from build123d import *

# Parameters (mm, degrees)
SKETCH_1_R          = 4
EXTRUDE_1_DEPTH     = 10
SKETCH_2_R          = 2.6
CUT_EXTRUDE_1_DEPTH = 10


with BuildPart() as part:
    # 草图1 → 凸台-拉伸1 (new body)
    with BuildSketch(Plane.XY):
        with BuildLine():
            Line((-27.5, -15), (27.5, -15))
            Line((27.5, -15), (27.5, -9.7))
            Line((27.5, -9.7), (15, -9.7))
            Line((15, -9.7), (15, 0))
            ThreePointArc((15, 0), (0, 15), (-15, 0))
            Line((-15, 0), (-15, -9.7))
            Line((-15, -9.7), (-27.5, -9.7))
            Line((-27.5, -9.7), (-27.5, -15))
        make_face()
        Circle(SKETCH_1_R, mode=Mode.SUBTRACT)
    extrude(amount=EXTRUDE_1_DEPTH)

    # 草图2 → 切除-拉伸1 (cut)
    with BuildSketch(Plane(origin=(0, -9.7, 0), x_dir=(1, 0, 0), z_dir=(0, 1, 0))):
        with Locations((21, -5)):
            Circle(SKETCH_2_R)
        with Locations((-21, -5)):
            Circle(SKETCH_2_R)
    extrude(amount=-CUT_EXTRUDE_1_DEPTH, mode=Mode.SUBTRACT)


solid = part.part
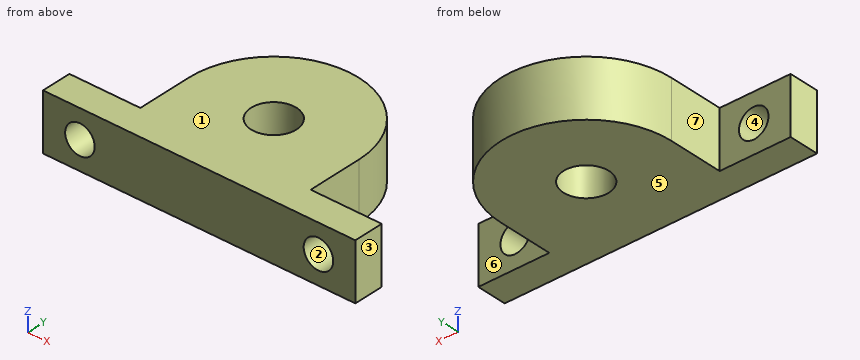
Here's how the part is built. I have some questions about the finished solid (model axes, mm). Face numbers are marked on the shaded views. A direction names the side the tool comes from. Give positions to 0.01 mm unless a question says otherwise; leave off trailing zeros. Order: outer loops, then holes, each group sorted by start corner. A loop starts at its lowest first (then second) coordinate and runs counter-clockwise, first axis right, second up. Notation, with made-up numbers: M 76,-1.5 L 81,-1.5 A7 ccw 81,8.5 Z; hole C -25,41 d3. An arc over 180 degrees is marked long. Answer as a JSON object with one key per item and string values. Group by question number.
1) Suppose I cut it at D-D, the plane y = -4.75. Write out the boundary of the cut face in (x, z), plus the area to 3 significant figures.
2) I'm going to push flat-ended pins straight in: pin 1 Ø5 at (y, z) = (-8, 2) entering from +X; pin 2 Ø2 at (y, z) = (-6, 6.5) entering from -X; pin 3 Ø6 at (x, z) = (9, 4) entering from +Y; pin 4 Ø3 at (y, z) = (9.5, 1) entering from +X. Where does each tip first touch, or does it pass through?
3) Please list where these lines run through material, in increasing order: L1, parallel to Z at x = -21, y = -11.1; L2, parallel to X at y = -11.95, z = 5; L3, parallel to Y at x = 0, z = 6.5. Write a range as [from, to].
4) Suppose I cut it at A-A, the plane z = 5. Write out the boundary of the cut face in (x, y), plus the area to 3 significant figures.
5) We'd pull the mould along X, two halves only. Please class the marked faces 1, 2, 3 and 4: pulls with the +X half, pulls with the -X half, needs draft (parallel to the pull), parting line crosses it, or undercut.
6) Suppose I cut it at B-B, the plane x = 21. Write out the boundary of the cut face in (y, z), plus the area to 3 significant figures.
7) On a 3-axis mill with a long thin cutter (end or side, diameter ignored), from which of +Z, -Z, +X, -X, +Y, -Y can I reach the whole of each face in a straight line? I mean the marked faces 5, 6 and 7. Say none if no direction works.
8) Suppose I cut it at C-C, the plane y = 2. Write out the boundary of the cut face in (x, z).
Results found:
{
 "1": {"outline": "M -15,0 L 15,0 L 15,10 L -15,10 Z", "area": "300 mm²"},
 "2": {"pin 1": "x = 27.5", "pin 2": "x = -15", "pin 3": "y = 13.75", "pin 4": "x = 12.69"},
 "3": {"L1": "[0, 2.4], [7.6, 10]", "L2": "[-27.5, -23.6], [-18.4, 18.4], [23.6, 27.5]", "L3": "[-15, -4], [4, 15]"},
 "4": {"outline": "M -27.5,-15 L -23.6,-15 L -23.6,-9.7 L -27.5,-9.7 Z; M -18.4,-15 L 18.4,-15 L 18.4,-9.7 L 15,-9.7 L 15,0 A15 ccw -15,0 L -15,-9.7 L -18.4,-9.7 Z; M 23.6,-15 L 27.5,-15 L 27.5,-9.7 L 23.6,-9.7 Z; hole C 0,0 d8", "area": "831 mm²"},
 "5": {"face 1": "needs draft", "face 2": "undercut", "face 3": "pulls with the +X half", "face 4": "undercut"},
 "6": {"outline": "M -15,0 L -9.7,0 L -9.7,2.4 L -15,2.4 Z; M -15,7.6 L -9.7,7.6 L -9.7,10 L -15,10 Z", "area": "25.4 mm²"},
 "7": {"face 5": "-Z, +X, -X, +Y, -Y", "face 6": "+Z, -Z, +X, +Y", "face 7": "+Z, -Z, -X, +Y"},
 "8": {"outline": "M -14.87,0 L -3.46,0 L -3.46,10 L -14.87,10 Z; M 3.46,0 L 14.87,0 L 14.87,10 L 3.46,10 Z"}
}
